Design review of the part built by this model. Coordinates are the model's own, in mm. Face numbers are marked on the shaded views. A direction names the side the tool comes from. Give positions to 0.01 mm unless a question says otherwise; leave off trailing zeros. Write each loop counter-clockwise with the first axis right and the second up, starting at its lowest first coordinate (ties: lowest second). Pieces come first, ordered by that corner, then holes. Notation, with made-up numbers: M 39.25,50 L 79.25,50 A34 cw 79.25,86 Z; hole C 3.5,-11.75 d8. An arc over 180 degrees is marked long. Use one line per item in the form item = value. Start each with the question number.
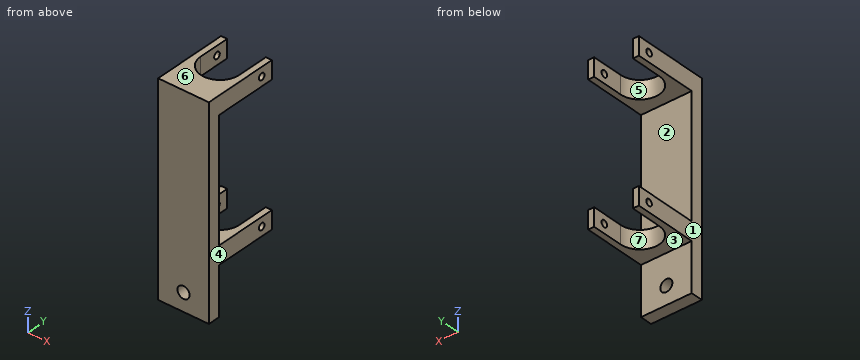
from build123d import *

# Parameters (mm, degrees)
F0_W      = 42
F0_H      = 52
F1_DEPTH  = 15
F3_DEPTH  = 50
F4_W      = 42
F4_H      = 10
F5_DEPTH  = 100
F6_W      = 42
F6_H      = 52
F7_DEPTH  = 15
F8_DEPTH  = 200
F9_W      = 42
F9_H      = 10
F10_DEPTH = 170
F11_R     = 5
F12_DEPTH = 25
F13_R     = 2.75
F14_DEPTH = 100
F15_W     = 10
F15_H     = 100
F16_DEPTH = 60


with BuildPart() as f1:
    # F0 (on Top) → F1 (new body)
    with BuildSketch(Plane.XY):
        Rectangle(F0_W, F0_H)
    extrude(amount=F1_DEPTH)

    # F2 (on face) → F3 (cut)
    with BuildSketch(Plane.XY.offset(15)):
        with BuildLine():
            Line((-16, 26), (-16, 0))
            ThreePointArc((-16, 0), (0, -16), (16, 0))
            Line((16, 0), (16, 26))
            Line((16, 26), (-16, 26))
        make_face()
    extrude(amount=-F3_DEPTH, mode=Mode.SUBTRACT)

    # F4 (on face) → F5 (join)
    with BuildSketch(Plane.XY.offset(15)):
        with Locations((0, -21)):
            Rectangle(F4_W, F4_H)
    extrude(amount=F5_DEPTH)

    # F6 (on face) → F7 (join)
    with BuildSketch(Plane.XY.offset(115)):
        Rectangle(F6_W, F6_H)
    extrude(amount=F7_DEPTH)

    # F2 (on face) → F8 (cut)
    with BuildSketch(Plane.XY.offset(15)):
        with BuildLine():
            Line((-16, 26), (-16, 0))
            ThreePointArc((-16, 0), (0, -16), (16, 0))
            Line((16, 0), (16, 26))
            Line((16, 26), (-16, 26))
        make_face()
    extrude(amount=F8_DEPTH, mode=Mode.SUBTRACT)

    # F9 (on face) → F10 (join)
    with BuildSketch(Plane.XY.offset(130)):
        with Locations((0, -31)):
            Rectangle(F9_W, F9_H)
    extrude(amount=-F10_DEPTH)

    # F11 (on face) → F12 (cut)
    with BuildSketch(Plane(origin=(0, -26, 0), x_dir=(-1, 0, 0), z_dir=(0, 1, 0))):
        with Locations((0, -25)):
            Circle(F11_R)
    extrude(amount=-F12_DEPTH, mode=Mode.SUBTRACT)

    # F13 (on face) → F14 (cut, symmetric)
    with BuildSketch(Plane(origin=(-21, 0, 0), x_dir=(0, -1, 0), z_dir=(-1, 0, 0))):
        with Locations((-16, 122.5)):
            Circle(F13_R)
        with Locations((-16, 7.5)):
            Circle(F13_R)
    extrude(amount=F14_DEPTH, both=True, mode=Mode.SUBTRACT)

    # F15 (on face) → F16 (cut)
    with BuildSketch(Plane.YZ.offset(21)):
        with Locations((-21, 65)):
            Rectangle(F15_W, F15_H)
    extrude(amount=-F16_DEPTH, mode=Mode.SUBTRACT)


solid = f1.part
1. Clearance check with flat-ended pins moving along their axes: pin 1 Ø21 at (x, y) = (5.5, -12.5) entering from -Z; pin 2 Ø6 at (x, z) = (0, -25) entering from +Y; pin 3 Ø3 at (x, z) = (6.5, 56.5) entering from +Y. State where each tip first meets the part, or that it passes through.
2. For the marked faces 1, 2 and 3, list the 3-axis set-ups (+Z, -Z, +X, -X, +Y, -Y) from which the entire face can be reached by the end or side of a thin tool; tool diameter is ignored.
3. We need section B-B (y = 22.5). State the section outline as (x, z) points.
4. To check wall thickness, follow L1, parallel to Z at x = -18.1, y = 16; L2, parallel to Z at x = -18, y = -4; L3, parallel to Z at x = 0, y = -28.5. State the ranges of each line that lie inside material, in increasing order.
5. We need section A-A (x = 0). State the section outline as (y, z) points, and give its area (3 significant figures).
6. We need section D-D (z = -25). State the section outline as (x, y) points.
7. We need section C-C (z = 122.5). State the section outline as (x, y) points.
8. Draft analysis for pull direction X (two halves, no side actions). For the marked faces 4, 5, 6 and 7, state which applies: pulls with the +X half, pulls with the -X half, needs draft (parallel to the pull), parting line crosses it, or undercut.
Answer block:
q1.pin_1 = 0
q1.pin_2 = through
q1.pin_3 = -26
q2.face_1 = +Z, -Z, -X, +Y, -Y
q2.face_2 = +X, -X, +Y
q2.face_3 = -Z, +X, -X, +Y
q3.outline = M -21,0 L -16,0 L -16,15 L -21,15 Z; M -21,115 L -16,115 L -16,130 L -21,130 Z; M 16,0 L 21,0 L 21,15 L 16,15 Z; M 16,115 L 21,115 L 21,130 L 16,130 Z
q4.L1 = 0 to 4.75, 10.25 to 15, 115 to 119.75, 125.25 to 130
q4.L2 = 0 to 15, 115 to 130
q4.L3 = -40 to -30, -20 to 130
q5.outline = M -36,-40 L -26,-40 L -26,-30 L -36,-30 Z; M -36,-20 L -26,-20 L -26,0 L -16,0 L -16,15 L -26,15 L -26,115 L -16,115 L -16,130 L -36,130 Z
q5.area = 1,900 mm^2
q6.outline = M -21,-36 L -5,-36 L -5,-26 L -21,-26 Z; M 5,-36 L 21,-36 L 21,-26 L 5,-26 Z
q7.outline = M -21,-36 L 21,-36 L 21,13.25 L 16,13.25 L 16,0 A16 cw -16,0 L -16,13.25 L -21,13.25 Z; M -21,18.75 L -16,18.75 L -16,26 L -21,26 Z; M 16,18.75 L 21,18.75 L 21,26 L 16,26 Z
q8.face_4 = pulls with the +X half
q8.face_5 = undercut
q8.face_6 = needs draft
q8.face_7 = undercut
